from build123d import *

# Parameters (mm, degrees)
SKETCH_W        = 150
SKETCH_H        = 100
PAD_DEPTH       = 40
SKETCH001_R     = 3.5
PAD001_DEPTH    = 5
SKETCH002_W     = 16
SKETCH002_H     = 31
POCKET_DEPTH    = 150
SKETCH003_W     = 126
SKETCH003_H     = 26
POCKET001_DEPTH = 100
POCKET002_DEPTH = 17
POCKET003_DEPTH = 18


with BuildPart() as part:
    # Sketch → Pad (new body)
    with BuildSketch(Plane.XY):
        Rectangle(SKETCH_W, SKETCH_H)
    extrude(amount=PAD_DEPTH)

    # Sketch001 (on Face5 of Pad) → Pad001 (join)
    with BuildSketch(Plane(origin=(0, 0, 0), x_dir=(1, 0, 0), z_dir=(0, 0, -1))):
        with Locations((67.5, 30)):
            Circle(SKETCH001_R)
        with Locations((67.5, -30)):
            Circle(SKETCH001_R)
        with Locations((-67.5, -30)):
            Circle(SKETCH001_R)
        with Locations((-67.5, 30)):
            Circle(SKETCH001_R)
    extrude(amount=PAD001_DEPTH)

    # Sketch002 (on Face3 of Pad001) → Pocket (cut)
    with BuildSketch(Plane.YZ.offset(75)):
        with Locations((42, 15.5)):
            Rectangle(SKETCH002_W, SKETCH002_H)
        with Locations((-42, 15.5)):
            Rectangle(SKETCH002_W, SKETCH002_H)
    extrude(amount=-POCKET_DEPTH, mode=Mode.SUBTRACT)

    # Sketch003 (on Face8 of Pocket) → Pocket001 (cut)
    with BuildSketch(Plane.XZ.offset(34)):
        with Locations((0, 13)):
            Rectangle(SKETCH003_W, SKETCH003_H)
    extrude(amount=-POCKET001_DEPTH, mode=Mode.SUBTRACT)

    # Sketch004 (on Face4 of Pocket001) → Pocket002 (cut)
    with BuildSketch(Plane.XY.offset(40)):
        with BuildLine():
            ThreePointArc((37.5, 22.5), (35, 20), (37.5, 17.5))
            Line((37.5, 17.5), (47.5, 17.5))
            ThreePointArc((47.5, 17.5), (50, 20), (47.5, 22.5))
            Line((47.5, 22.5), (37.5, 22.5))
        make_face()
        with BuildLine():
            ThreePointArc((45, 12.5), (42.5, 10), (45, 7.5))
            Line((45, 7.5), (55, 7.5))
            ThreePointArc((55, 7.5), (57.5, 10), (55, 12.5))
            Line((55, 12.5), (45, 12.5))
        make_face()
        with BuildLine():
            ThreePointArc((27.5, 32.5), (25, 30), (27.5, 27.5))
            Line((27.5, 27.5), (37.5, 27.5))
            ThreePointArc((37.5, 27.5), (40, 30), (37.5, 32.5))
            Line((37.5, 32.5), (27.5, 32.5))
        make_face()
        with BuildLine():
            ThreePointArc((20, 22.5), (17.5, 20), (20, 17.5))
            Line((20, 17.5), (30, 17.5))
            ThreePointArc((30, 17.5), (32.5, 20), (30, 22.5))
            Line((30, 22.5), (20, 22.5))
        make_face()
        with BuildLine():
            ThreePointArc((10, 12.5), (7.5, 10), (10, 7.5))
            Line((10, 7.5), (20, 7.5))
            ThreePointArc((20, 7.5), (22.5, 10), (20, 12.5))
            Line((20, 12.5), (10, 12.5))
        make_face()
        with BuildLine():
            ThreePointArc((27.5, 12.5), (25, 10), (27.5, 7.5))
            Line((27.5, 7.5), (37.5, 7.5))
            ThreePointArc((37.5, 7.5), (40, 10), (37.5, 12.5))
            Line((37.5, 12.5), (27.5, 12.5))
        make_face()
    pocket002 = extrude(amount=-POCKET002_DEPTH, mode=Mode.SUBTRACT)

    # Sketch005 (on Face4 of Pocket002) → Pocket003 (cut)
    with BuildSketch(Plane.XY.offset(40)):
        with BuildLine():
            ThreePointArc((10.816809, -7.5), (8.316809, -10), (10.816809, -12.5))
            Line((10.816809, -12.5), (20.816809, -12.5))
            ThreePointArc((20.816809, -12.5), (23.316809, -10), (20.816809, -7.5))
            Line((20.816809, -7.5), (10.816809, -7.5))
        make_face()
        with BuildLine():
            ThreePointArc((28.316809, -7.5), (25.816809, -10), (28.316809, -12.5))
            Line((28.316809, -12.5), (38.316809, -12.5))
            ThreePointArc((38.316809, -12.5), (40.816809, -10), (38.316809, -7.5))
            Line((38.316809, -7.5), (28.316809, -7.5))
        make_face()
        with BuildLine():
            ThreePointArc((45.816809, -7.5), (43.316809, -10), (45.816809, -12.5))
            Line((45.816809, -12.5), (55.816809, -12.5))
            ThreePointArc((55.816809, -12.5), (58.316809, -10), (55.816809, -7.5))
            Line((55.816809, -7.5), (45.816809, -7.5))
        make_face()
        with BuildLine():
            ThreePointArc((20, -17.5), (17.5, -20), (20, -22.5))
            Line((20, -22.5), (30, -22.5))
            ThreePointArc((30, -22.5), (32.5, -20), (30, -17.5))
            Line((30, -17.5), (20, -17.5))
        make_face()
        with BuildLine():
            ThreePointArc((37.5, -17.5), (35, -20), (37.5, -22.5))
            Line((37.5, -22.5), (47.5, -22.5))
            ThreePointArc((47.5, -22.5), (50, -20), (47.5, -17.5))
            Line((47.5, -17.5), (37.5, -17.5))
        make_face()
        with BuildLine():
            ThreePointArc((28.316809, -27.5), (25.816809, -30), (28.316809, -32.5))
            Line((28.316809, -32.5), (38.316809, -32.5))
            ThreePointArc((38.316809, -32.5), (40.816809, -30), (38.316809, -27.5))
            Line((38.316809, -27.5), (28.316809, -27.5))
        make_face()
    pocket003 = extrude(amount=-POCKET003_DEPTH, mode=Mode.SUBTRACT)

    # Mirrored: Pocket002 across Sketch004 V_Axis
    add(pocket002.mirror(Plane(origin=(0, 0, 40), x_dir=(0, 0, 1), z_dir=(1, 0, 0))), mode=Mode.SUBTRACT)

    # Mirrored001: Pocket003 across Sketch005 V_Axis
    add(pocket003.mirror(Plane(origin=(0, 0, 40), x_dir=(0, 0, 1), z_dir=(1, 0, 0))), mode=Mode.SUBTRACT)


solid = part.part
Verification items for the finished model (mm, model axes). A direction names the side the tool comes from. Round coordinates to 2 decimals unless told otherwise and drop trailing zeros. Loops run counter-clockwise (first coordinate to the right, second up) from the corner with the lowest first, then second, coordinate; pieces in that order, holes last. Notation, with made-up numbers: (46, 38) - (89, 38) arc R15 cw to (89, 63) - close; hole circle Ø5 at (-30.5, -8.5). An arc over 180 degrees is marked (long way). Answer in a Markdown table with one row per item. Add a question column.
Q1. Section check C-C on z = 20. Enter the section's corners in (x, y), plus the area to 3 significant figures.
Q2. Section check B-B on y = -30. Enter the section's corners in (x, z).
Q3. Section check D-D on y = -10. State how many separate pieces and enclosed holes the cut face has, plus the area to 3 significant figures.
Q4. Gauge pin test, flat ends, axial feed: pin 1 (1.5 mm diameter, centred on x = 52, z = 26, fed in from +Y); pin 2 (12 mm diameter, centred on x = -29.5, y = -23, fed in from -Z). Record the tip position at first contact, or that the pin passes through.
Q5. Tool access check on faces 1 (the face through (-16, -7.5, 33)), 2 (the face through (64.92, -32.365, -2.465)). Record the directions out of +Z, -Z, +X, -X, +Y, -Y that give a thin tool (end or side, any length) a straight path to the whole face; none if there is none.
Q6. Material ranges on line 1 (Y direction, x = 23.5, z = 28); line 2 (X direction, y = 3.5, z = 18); line 3 (Z direction, x = 45, y = 13), recorded low to high.
Q7. Section check A-A on y = 20. Enter the section's corners in (x, z), plus the area to 3 significant figures.
Found:
| question | item | result |
|---|---|---|
| 1 | outline | (-75, -34) - (-63, -34) - (-63, 34) - (-75, 34) - close; (63, -34) - (75, -34) - (75, 34) - (63, 34) - close |
| 1 | area | 1,630 mm² |
| 2 | outline | (-75, 0) - (-71, 0) - (-71, -5) - (-64, -5) - (-64, 0) - (-63, 0) - (-63, 26) - (-40.82, 26) - (-40.82, 40) - (-75, 40) - close; (-25.82, 26) - (25.82, 26) - (25.82, 40) - (-25.82, 40) - close; (40.82, 26) - (63, 26) - (63, 0) - (64, 0) - (64, -5) - (71, -5) - (71, 0) - (75, 0) - (75, 40) - (40.82, 40) - close |
| 3 | separate pieces | 7 |
| 3 | enclosed holes | 0 |
| 3 | area | 1,460 mm² |
| 4 | pin 1 | stops at y = 34 |
| 4 | pin 2 | stops at z = 26 |
| 5 | face 1 | +Z, -Z |
| 5 | face 2 | -Z |
| 6 | line 1 | y = -34 to -22.5, -17.5 to 17.5, 22.5 to 34 |
| 6 | line 2 | x = -75 to -63, 63 to 75 |
| 6 | line 3 | z = 26 to 40 |
| 7 | outline | (-75, 0) - (-63, 0) - (-63, 26) - (-50, 26) - (-50, 40) - (-75, 40) - close; (-35, 26) - (-32.5, 26) - (-32.5, 40) - (-35, 40) - close; (-17.5, 26) - (17.5, 26) - (17.5, 40) - (-17.5, 40) - close; (32.5, 26) - (35, 26) - (35, 40) - (32.5, 40) - close; (50, 26) - (63, 26) - (63, 0) - (75, 0) - (75, 40) - (50, 40) - close |
| 7 | area | 1,880 mm² |
